Design review of the part built by this model. Coordinates are the model's own, in mm. A direction names the side the tool comes from. Coordinates: 2 decimals unless noted, no trailing zeros. Order: outer loops, then holes, each group sorted by start corner. A loop starts at its lowest first (then second) coordinate and runs counter-clockwise, first axis right, second up. Notation, with made-up numbers: M 27,56.25 L 70,56.25 A17 cw 70,71.25 Z; hole C -30.5,-15.5 d9. An arc over 180 degrees is marked long. Use CSV: the item, a comma, the result in double quotes.
```python
from build123d import *

# Parameters (mm, degrees)
EXTRUDE_1_DEPTH = 3
SKETCH_2_W      = 23.4
SKETCH_2_H      = 15.4
EXTRUDE_2_DEPTH = 3
SKETCH_4_W      = 23.4
SKETCH_4_H      = 15.4
SKETCH_4_W_2    = 20.4
SKETCH_4_H_2    = 12.4
EXTRUDE_4_DEPTH = 16.4


with BuildPart() as part:
    # 草图1 → 凸台-拉伸1 (new body)
    with BuildSketch(Plane(origin=(0, 0, 0), x_dir=(1, 0, 0), z_dir=(0, 1, 0))):
        with BuildLine():
            Line((7, 5), (25.5, 5))
            ThreePointArc((25.5, 5), (26.914213562, 4.414213562), (27.5, 3))
            Line((27.5, 3), (27.5, -3))
            ThreePointArc((27.5, -3), (26.914213562, -4.414213562), (25.5, -5))
            Line((25.5, -5), (7, -5))
            ThreePointArc((7, -5), (5.585786438, -5.585786438), (5, -7))
            Line((5, -7), (5, -25.5))
            ThreePointArc((5, -25.5), (4.414213562, -26.914213562), (3, -27.5))
            Line((3, -27.5), (-3, -27.5))
            ThreePointArc((-3, -27.5), (-4.414213562, -26.914213562), (-5, -25.5))
            Line((-5, -25.5), (-5, -7))
            ThreePointArc((-5, -7), (-5.585786438, -5.585786438), (-7, -5))
            Line((-7, -5), (-25.5, -5))
            ThreePointArc((-25.5, -5), (-26.914213562, -4.414213562), (-27.5, -3))
            Line((-27.5, -3), (-27.5, 3))
            ThreePointArc((-27.5, 3), (-26.914213562, 4.414213562), (-25.5, 5))
            Line((-25.5, 5), (-7, 5))
            ThreePointArc((-7, 5), (-5.585786438, 5.585786438), (-5, 7))
            Line((-5, 7), (-5, 25.5))
            ThreePointArc((-5, 25.5), (-4.414213562, 26.914213562), (-3, 27.5))
            Line((-3, 27.5), (3, 27.5))
            ThreePointArc((3, 27.5), (4.414213562, 26.914213562), (5, 25.5))
            Line((5, 25.5), (5, 7))
            ThreePointArc((5, 7), (5.585786438, 5.585786438), (7, 5))
        make_face()
    extrude(amount=EXTRUDE_1_DEPTH)

    # 草图2 → 凸台-拉伸2 (add)
    with BuildSketch(Plane.XZ):
        Rectangle(SKETCH_2_W, SKETCH_2_H)
    extrude(amount=EXTRUDE_2_DEPTH)

    # 草图4 → 凸台-拉伸4 (add)
    with BuildSketch(Plane.XZ.offset(3)):
        Rectangle(SKETCH_4_W, SKETCH_4_H)
        Rectangle(SKETCH_4_W_2, SKETCH_4_H_2, mode=Mode.SUBTRACT)
    extrude(amount=EXTRUDE_4_DEPTH)


solid = part.part
```
(1) Add section A-A on y = -4.75. State the section outline as (x, z) points.
The answers:
outline,"M -11.7,-7.7 L 11.7,-7.7 L 11.7,7.7 L -11.7,7.7 Z; hole M -10.2,-6.2 L 10.2,-6.2 L 10.2,6.2 L -10.2,6.2 Z"
(2) Add section C-C on z = -1. State the section outline as (x, y) points, and give its area (3 significant figures).
The answers:
outline,"M -27.5,0 L -11.7,0 L -11.7,-19.4 L -10.2,-19.4 L -10.2,-3 L 10.2,-3 L 10.2,-19.4 L 11.7,-19.4 L 11.7,0 L 27.5,0 L 27.5,3 L -27.5,3 Z"
area,"284 mm2"
(3) Wall thickness on probe 1 along X at (y, z) = (-15.25, 5.5); probe 2 along Z at (x, y) = (-2, -14.75); probe 3 along Y at (x, z) = (-17, 0): over which ranges is each line inside the solid? List them lowest first.
The answers:
probe 1,"x = -11.7 to -10.2, 10.2 to 11.7"
probe 2,"z = -7.7 to -6.2, 6.2 to 7.7"
probe 3,"y = 0 to 3"
(4) Clearance check with flat-ended pins moving along their axes: P1, Ø5, axis at x = 7.5, y = -5.5, coming from the -Z side; P2, Ø0.9, axis at y = 1.5, z = 16, coming from the -X side; P3, Ø2, axis at x = -9, z = -7, coming from the +Y side; P4, Ø12, axis at x = 16, z = -21, coming from the +Y side (3 decimals). State where each tip first meets the part, or that it passes through.
The answers:
P1,"stops at z = -7.7"
P2,"stops at x = -5"
P3,"stops at y = 0"
P4,"passes through"
(5) The part is to be moulded in two halves that separate along Z. For faces 1 (the face through (20, 0, 0)), 2 (the face through (5.57, 1.48, -5.6)), 3 (the face through (16, 1, 5)), 4 (the face through (0, -3, 0)), say which applies: pulls with the +Z half, pulls with the -Z half, needs draft (parallel to the pull), parting line crosses it, or undercut.
The answers:
face 1,"needs draft"
face 2,"pulls with the -Z half"
face 3,"pulls with the +Z half"
face 4,"undercut"
(6) Add section B-B on x = 9.5. State the section outline as (y, z) points, and give its area (3 significant figures).
The answers:
outline,"M -19.4,-7.7 L 0,-7.7 L 0,-5 L 3,-5 L 3,5 L 0,5 L 0,7.7 L -19.4,7.7 L -19.4,6.2 L -3,6.2 L -3,-6.2 L -19.4,-6.2 Z"
area,"125 mm2"
(7) Add section D-D on y = -1.25. State the section outline as (x, z) points, and give its area (3 significant figures).
The answers:
outline,"M -11.7,-7.7 L 11.7,-7.7 L 11.7,7.7 L -11.7,7.7 Z"
area,"360 mm2"
(8) For faces 5 (the face through (0, -10, 7.7)), 6 (the face through (8, 0, -6)), 7 (the face through (8, 0, 6)), 8 (the face through (-16, 1, -5)), list the 3-axis set-ups (+Z, -Z, +X, -X, +Y, -Y) from which the entire face can be reached by the end or side of a thin tool; tool diameter is ignored.
The answers:
face 5,"+Z, +X, -X, -Y"
face 6,"-Z, +X, +Y"
face 7,"+Z, +X, +Y"
face 8,"-Z, -X, +Y"
